Check sheet for the modelled part. Datum: model origin and axes. Units: mm. Face numbers are marked on the shaded views. A direction names the side the tool comes from. Coordinates: 2 decimals unless noted, no trailing zeros. Loops run counter-clockwise (first coordinate to the right, second up) from the corner with the lowest first, then second, coordinate; pieces in that order, holes last. Notation, with made-up numbers: (8, 22.25) - (52, 22.25) arc R7 ccw to (52, 32.25) - close; hole circle Ø1 at (29.5, -23). An arc over 180 degrees is marked (long way). Use a Markdown table: item, result. Add a question column.
1) Go/stop test with flat-tipped pins: P1, Ø5.5, axis at x = 9, z = -5.5, coming from the +Y side; P2, Ø10, axis at x = 8, z = 9.5, coming from the -Y side; P3, Ø5.5, axis at x = 12.5, y = -4, coming from the +Z side; P4, Ø3.5, axis at x = 7.5, y = 44, coming from the -Z side. Record where each tip stops, or that it passes through.
2) Sectioned sample at C-C, the plane y = -1. Enter the section's corners in (x, z).
3) Sectioned sample at A-A, the plane x = 14. Enter the section's corners in (y, z), then the cut area to 3 significant figures.
4) Sectioned sample at B-B, the plane z = 16.5. Enter the section's corners in (x, y), then the cut area to 3 significant figures.
5) Tool access check on the marked faces 1, 2 and 3. Record the directions out of +Z, -Z, +X, -X, +Y, -Y that give a thin tool (end or side, any length) a straight path to the whole face; none if there is none.
6) Thickness scan on line 1 (Y direction, x = 11.75, z = 25); line 2 (Z direction, x = 12.5, y = -3). Record the ranges inside material, lowest first.
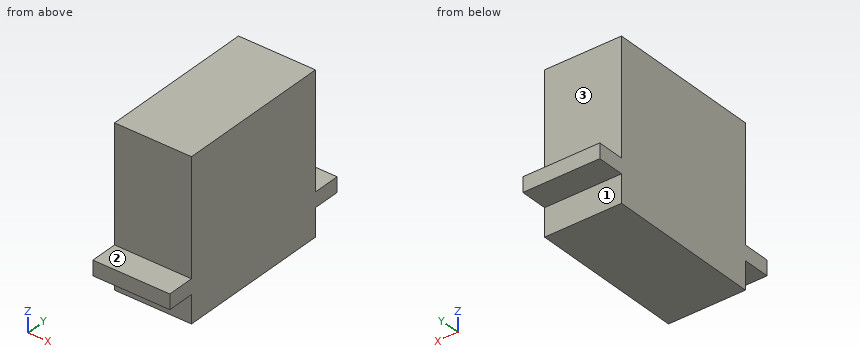
Autodesk Inventor part; units mm, degrees
ref_plane "YZ Plane" through (0, 0, 0) normal (1, 0, 0) x (0, 1, 0)
ref_plane "XZ Plane" through (0, 0, 0) normal (0, 1, 0) x (-1, 0, 0)
ref_plane "XY Plane" through (0, 0, 0) normal (0, 0, 1) x (1, 0, 0)
sketch "Sketch1" plane through (0, 0, 0) normal (0, 0, 1) x (1, 0, 0)
  line L0 (0, 0) -> (19.7866, 0)
  line L1 (19.7866, 0) -> (19.7866, 40.2336)
  line L2 (19.7866, 40.2336) -> (0, 40.2336)
  line L3 (0, 40.2336) -> (0, 0)
  line L4 (0, 0) -> (19.7866, 0)
  line L5 (19.7866, 0) -> (19.7866, -7.0358)
  line L6 (19.7866, -7.0358) -> (0, -7.0358)
  line L7 (0, -7.0358) -> (0, 0)
  line L8 (19.7866, 20.1168) -> (0, 20.1168) construction
  line L9 (19.7866, 40.2336) -> (19.7866, 47.2694)
  line L10 (19.7866, 47.2694) -> (0, 47.2694)
  line L11 (0, 47.2694) -> (0, 40.2336)
  dimension "d0" = 19.7866
  dimension "d1" = 40.2336
  dimension "d2" = 7.0358
extrude "Extrusion1" add sketch "Sketch1" along normal blind 29.591 contours L3 L2 L1 L0
extrude "Extrusion2" add sketch "Sketch1" against normal blind 3.81 contours L0 L5 L6 L7 | L11 L10 L9 L2
extrude "Extrusion3" add sketch "Sketch1" against normal blind 10.9601 contours L3 L2 L1 L0
properties part number "ServoSimplified"
Solved:
| question | item | result |
|---|---|---|
| 1 | P1 | stops at y = 47.27 |
| 1 | P2 | stops at y = 0 |
| 1 | P3 | stops at z = 0 |
| 1 | P4 | stops at z = -3.81 |
| 2 | outline | (0, -3.81) - (19.79, -3.81) - (19.79, 0) - (0, 0) - close |
| 3 | outline | (-7.04, -3.81) - (0, -3.81) - (0, -10.96) - (40.23, -10.96) - (40.23, -3.81) - (47.27, -3.81) - (47.27, 0) - (40.23, 0) - (40.23, 29.59) - (0, 29.59) - (0, 0) - (-7.04, 0) - close |
| 3 | area | 1,690 mm2 |
| 4 | outline | (0, 0) - (19.79, 0) - (19.79, 40.23) - (0, 40.23) - close |
| 4 | area | 796 mm2 |
| 5 | face 1 | -Z, +X, -X, +Y |
| 5 | face 2 | +Z, +X, -X, -Y |
| 5 | face 3 | +Z, +X, -X, +Y |
| 6 | line 1 | y = 0 to 40.23 |
| 6 | line 2 | z = -3.81 to 0 |
